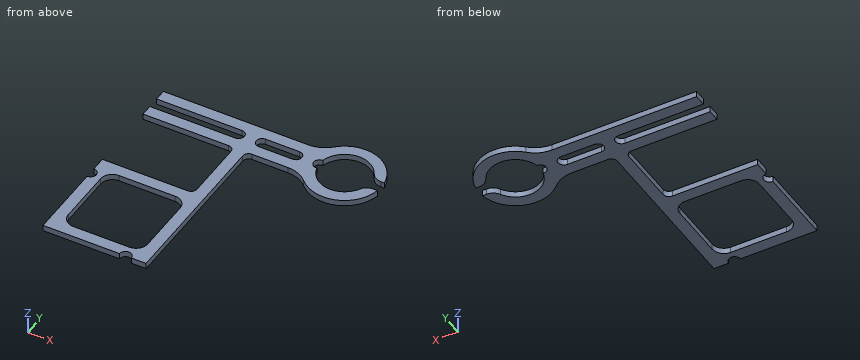
```python
from build123d import *

# Parameters (mm, degrees)
SKETCH_W    = 13.5
SKETCH_H    = 13.5
PAD_DEPTH   = 1
FILLET_R    = 2
FILLET001_R = 5
FILLET002_R = 1
FILLET003_R = 2


with BuildPart() as fillet003:
    # Sketch → Pad (new body)
    with BuildSketch(Plane.XY):
        with BuildLine():
            Line((0, 35.5), (-27.017072, 35.5))
            ThreePointArc((-27.017072, 35.5), (-33.557279, 38.659924), (-38.669481, 33.5))
            Line((-38.669481, 33.5), (-36.75, 33.5))
            ThreePointArc((-28.25, 33.5), (-32.5, 36.866062), (-36.75, 33.5))
            ThreePointArc((-28.367647, 31.506945), (-27.251738, 32.441074), (-28.25, 33.5))
            ThreePointArc((-36.630678, 31.5), (-32.496428, 28.250002), (-28.367647, 31.506945))
            Line((-38.669481, 31.5), (-36.630678, 31.5))
            ThreePointArc((-38.669481, 31.5), (-33.557279, 26.340076), (-27.017072, 29.5))
            Line((-27.017072, 29.5), (-17.5, 29.5))
            Line((-17.5, 29.5), (-17.5, 0))
            Line((-17.5, 0), (-15, 0))
            ThreePointArc((-13, 0), (-14, 1), (-15, 0))
            Line((0, 0), (-13, 0))
            Line((0, 13), (0, 0))
            ThreePointArc((0, 15), (-1, 14), (0, 13))
            Line((0, 17.5), (0, 15))
            Line((0, 17.5), (-15.5, 17.5))
            Line((-15.5, 17.5), (-15.5, 29.5))
            Line((-15.5, 29.5), (0, 29.5))
            Line((0, 29.5), (0, 31.5))
            Line((-14.5, 31.5), (0, 31.5))
            ThreePointArc((-14.5, 33.5), (-15.5, 32.5), (-14.5, 31.5))
            Line((-14.5, 33.5), (0, 33.5))
            Line((0, 33.5), (0, 35.5))
        make_face()
        with Locations((-8.75, 8.75)):
            Rectangle(SKETCH_W, SKETCH_H, mode=Mode.SUBTRACT)
        with BuildLine():
            ThreePointArc((-24.25, 33.5), (-25.25, 32.5), (-24.25, 31.5))
            Line((-24.25, 31.5), (-18.5, 31.5))
            ThreePointArc((-18.5, 31.5), (-17.5, 32.5), (-18.5, 33.5))
            Line((-24.25, 33.5), (-18.5, 33.5))
        make_face(mode=Mode.SUBTRACT)
    extrude(amount=PAD_DEPTH)

    # Fillet
    fillet_edges = [fillet003.edges().sort_by_distance(p)[0] for p in [
        (-36.75, 33.5, 0.5),
        (-36.630678, 31.5, 0.5),
    ]]
    fillet(fillet_edges, radius=FILLET_R)

    # Fillet001
    fillet001_edges = [fillet003.edges().sort_by_distance(p)[0] for p in [
        (-27.017072, 29.5, 0.5),
        (-27.017072, 35.5, 0.5),
    ]]
    fillet(fillet001_edges, radius=FILLET001_R)

    # Fillet002
    fillet002_edges = [fillet003.edges().sort_by_distance(p)[0] for p in [
        (-15.5, 17.5, 0.5),
        (-15.5, 29.5, 0.5),
        (-17.5, 29.5, 0.5),
    ]]
    fillet(fillet002_edges, radius=FILLET002_R)

    # Fillet003
    fillet003_edges = [fillet003.edges().sort_by_distance(p)[0] for p in [
        (-15.5, 15.5, 0.5),
        (-2, 15.5, 0.5),
        (-2, 2, 0.5),
        (-15.5, 2, 0.5),
    ]]
    fillet(fillet003_edges, radius=FILLET003_R)


with BuildPart() as part_mirroring:
    # Part__Mirroring: instance of Fillet003
    add(fillet003.part.mirror(Plane(origin=(0, 0, 0), x_dir=(1, 0, 0), z_dir=(0, 1, 0))))


with BuildPart() as part_mirroring001:
    # Part__Mirroring001: instance of Part__Mirroring
    add(part_mirroring.part.mirror(Plane(origin=(0, 0, 0), x_dir=(0, -1, 0), z_dir=(1, 0, 0))))


with BuildPart() as part_mirroring002:
    # Part__Mirroring002: instance of Part__Mirroring001
    add(part_mirroring001.part.mirror(Plane(origin=(0, 0, 0), x_dir=(1, 0, 0), z_dir=(0, 1, 0))))


solid = part_mirroring002.part
```
Build history of the part. All positions in model axes, mm. Round coordinates to 2 decimals unless told otherwise and drop trailing zeros. Write each loop counter-clockwise with the first axis right and the second up, starting at its lowest first coordinate (ties: lowest second). Pieces come first, ordered by that corner, then holes.
1) Band-saw the part on A-A, the plane x = 6. List the corners of the cut face in (y, z), and give its area (3 significant figures).
2) Band-saw the part on D-D, the plane z = 0.7. Give the number of separate pieces and of enclosed holes in the cut face, and give its area (3 significant figures).
3) Drill centre lines: probe 1 along Y at (x, z) = (9.5, 0.7); probe 2 along X at (y, z) = (8, 0.45); probe 3 along Y at (x, z) = (2.5, 0.2). Where is each one in solid material? Low to high.
4) Band-saw the part on B-B, the plane y = 11. List the corners of the cut face in (x, z).
5) Pin check, flat tips, straight feed: pin 1 (10 mm diameter, centred on x = 27, y = 23.5, fed in from +Z); pin 2 (0.5 mm diameter, centred on y = 7.5, z = 0.5, fed in from +X). Stop position of each tip, or through.
6) Band-saw the part on C-C, the plane x = 20. List the corners of the cut face in (y, z).
Ans:
1. outline: (0, 0) - (2, 0) - (2, 1) - (0, 1) - close; (15.5, 0) - (17.5, 0) - (17.5, 1) - (15.5, 1) - close; (29.5, 0) - (31.5, 0) - (31.5, 1) - (29.5, 1) - close; (33.5, 0) - (35.5, 0) - (35.5, 1) - (33.5, 1) - close
1. area: 8.00 mm2
2. separate pieces: 1
2. enclosed holes: 2
2. area: 323 mm2
3. probe 1: y = 0 to 2, 15.5 to 17.5, 29.5 to 31.5, 33.5 to 35.5
3. probe 2: x = 0 to 2, 15.5 to 17.5
3. probe 3: y = 0 to 2.68, 14.82 to 17.5, 29.5 to 31.5, 33.5 to 35.5
4. outline: (0, 0) - (2, 0) - (2, 1) - (0, 1) - close; (15.5, 0) - (17.5, 0) - (17.5, 1) - (15.5, 1) - close
5. pin 1: stops at z = 1
5. pin 2: stops at x = 17.5
6. outline: (29.5, 0) - (31.5, 0) - (31.5, 1) - (29.5, 1) - close; (33.5, 0) - (35.5, 0) - (35.5, 1) - (33.5, 1) - close
